The model under review builds one solid part; all positions refer to its coordinate system, in mm. Coordinates: 2 decimals unless noted, no trailing zeros. Order: outer loops, then holes, each group sorted by start corner. A loop starts at its lowest first (then second) coordinate and runs counter-clockwise, first axis right, second up.
```python
from build123d import *

# Parameters (mm, degrees)
SKETCH1_W           = 55.928846154
SKETCH1_H           = 3.175
SKETCH1_W_2         = 3.175
SKETCH1_W_3         = 59.103846154
SKETCH1_H_2         = 26.307142857
SKETCH1_H_3         = 26.307142858
BOSS_EXTRUDE1_DEPTH = 6.35
SKETCH2_W           = 3.175
SKETCH2_H           = 12.7
CUT_EXTRUDE1_DEPTH  = 396.105756412
SKETCH3_W           = 59.103846153
SKETCH3_H           = 3.175
SKETCH3_W_2         = 59.103846154
SKETCH3_W_3         = 3.175
SKETCH3_H_2         = 26.307142857
BOSS_EXTRUDE2_DEPTH = 6.35


with BuildPart() as part:
    # Sketch1 → Boss-Extrude1 (new body)
    with BuildSketch(Plane(origin=(0, 0, 0), x_dir=(1, 0, 0), z_dir=(0, 1, 0))):
        Polygon((0, -88.9), (0, 88.9), (-29.551923077, 88.9), (-88.655769231, 88.9), (-147.759615385, 88.9), (-206.863461538, 88.9), (-265.967307692, 88.9), (-325.071153846, 88.9), (-381, 88.9), (-381, 65.767857143), (-381, 39.460714286), (-381, 13.153571429), (-381, -13.153571429), (-381, -39.460714286), (-381, -65.767857143), (-381, -88.9), (-325.071153846, -88.9), (-265.967307692, -88.9), (-206.863461538, -88.9), (-147.759615385, -88.9), (-88.655769231, -88.9), (-29.551923077, -88.9), align=None)
        Polygon((29.551923077, 88.9), (0, 88.9), (0, -88.9), (29.551923077, -88.9), (88.655769231, -88.9), (147.759615385, -88.9), (206.863461538, -88.9), (265.967307692, -88.9), (325.071153846, -88.9), (381, -88.9), (381, -65.767857143), (381, -39.460714286), (381, -13.153571429), (381, 13.153571429), (381, 39.460714286), (381, 65.767857143), (381, 88.9), (325.071153846, 88.9), (265.967307692, 88.9), (206.863461538, 88.9), (147.759615385, 88.9), (88.655769231, 88.9), align=None)
        with Locations((-353.035576923, -90.4875)):
            Rectangle(SKETCH1_W, SKETCH1_H)
        with Locations((-382.5875, -90.4875)):
            Rectangle(SKETCH1_W_2, SKETCH1_H)
        with Locations((-236.415384615, -90.4875)):
            Rectangle(SKETCH1_W_3, SKETCH1_H)
        with Locations((-382.5875, -52.614285714)):
            Rectangle(SKETCH1_W_2, SKETCH1_H_2)
        with Locations((-118.207692308, -90.4875)):
            Rectangle(SKETCH1_W_3, SKETCH1_H)
        with Locations((-382.5875, 0)):
            Rectangle(SKETCH1_W_2, SKETCH1_H_3)
        with Locations((-382.5875, 52.614285714)):
            Rectangle(SKETCH1_W_2, SKETCH1_H_2)
        with Locations((-382.5875, 90.4875)):
            Rectangle(SKETCH1_W_2, SKETCH1_H)
        with Locations((-353.035576923, 90.4875)):
            Rectangle(SKETCH1_W, SKETCH1_H)
        with Locations((-236.415384615, 90.4875)):
            Rectangle(SKETCH1_W_3, SKETCH1_H)
        with Locations((-118.207692308, 90.4875)):
            Rectangle(SKETCH1_W_3, SKETCH1_H)
        Polygon((-29.551923077, 88.9), (0, 88.9), (29.551923077, 88.9), (29.551923077, 92.075), (-29.551923077, 92.075), align=None)
        with Locations((118.207692308, 90.4875)):
            Rectangle(SKETCH1_W_3, SKETCH1_H)
        Polygon((29.551923077, -88.9), (0, -88.9), (-29.551923077, -88.9), (-29.551923077, -92.075), (29.551923077, -92.075), align=None)
        with Locations((118.207692308, -90.4875)):
            Rectangle(SKETCH1_W_3, SKETCH1_H)
        with Locations((236.415384615, -90.4875)):
            Rectangle(SKETCH1_W_3, SKETCH1_H)
        with Locations((236.415384615, 90.4875)):
            Rectangle(SKETCH1_W_3, SKETCH1_H)
        with Locations((382.5875, 90.4875)):
            Rectangle(SKETCH1_W_2, SKETCH1_H)
        with Locations((382.5875, 52.614285714)):
            Rectangle(SKETCH1_W_2, SKETCH1_H_2)
        with Locations((382.5875, 0)):
            Rectangle(SKETCH1_W_2, SKETCH1_H_3)
        with Locations((382.5875, -52.614285714)):
            Rectangle(SKETCH1_W_2, SKETCH1_H_2)
        with Locations((382.5875, -90.4875)):
            Rectangle(SKETCH1_W_2, SKETCH1_H)
        with Locations((354.623076923, -90.4875)):
            Rectangle(SKETCH1_W_3, SKETCH1_H)
        with Locations((354.623076923, 90.4875)):
            Rectangle(SKETCH1_W_3, SKETCH1_H)
    extrude(amount=BOSS_EXTRUDE1_DEPTH)

    # Sketch2 → Cut-Extrude1 (cut, through all)
    with BuildSketch(Plane(origin=(0, 6.35, 0), x_dir=(1, 0, 0), z_dir=(0, 1, 0))):
        with Locations((-123.03125, 82.55)):
            Rectangle(SKETCH2_W, SKETCH2_H)
        with Locations((-123.03125, -82.55)):
            Rectangle(SKETCH2_W, SKETCH2_H)
        with Locations((130.96875, 82.55)):
            Rectangle(SKETCH2_W, SKETCH2_H)
        with Locations((130.96875, -82.55)):
            Rectangle(SKETCH2_W, SKETCH2_H)
    extrude(amount=-CUT_EXTRUDE1_DEPTH, mode=Mode.SUBTRACT)

    # Sketch3 → Boss-Extrude2 (add)
    with BuildSketch(Plane(origin=(0, 6.35, 0), x_dir=(1, 0, 0), z_dir=(0, 1, 0))):
        with Locations((-177.311538462, -90.4875)):
            Rectangle(SKETCH3_W, SKETCH3_H)
        with Locations((-59.103846154, -90.4875)):
            Rectangle(SKETCH3_W_2, SKETCH3_H)
        with Locations((59.103846154, -90.4875)):
            Rectangle(SKETCH3_W_2, SKETCH3_H)
        with Locations((177.311538462, -90.4875)):
            Rectangle(SKETCH3_W, SKETCH3_H)
        with Locations((382.5875, -26.307142858)):
            Rectangle(SKETCH3_W_3, SKETCH3_H_2)
        with Locations((382.5875, 26.307142858)):
            Rectangle(SKETCH3_W_3, SKETCH3_H_2)
        with Locations((-382.5875, -26.307142858)):
            Rectangle(SKETCH3_W_3, SKETCH3_H_2)
        with Locations((-382.5875, 26.307142858)):
            Rectangle(SKETCH3_W_3, SKETCH3_H_2)
        with Locations((-177.311538462, 90.4875)):
            Rectangle(SKETCH3_W, SKETCH3_H)
        with Locations((-59.103846154, 90.4875)):
            Rectangle(SKETCH3_W_2, SKETCH3_H)
        with Locations((59.103846154, 90.4875)):
            Rectangle(SKETCH3_W_2, SKETCH3_H)
        with Locations((177.311538462, 90.4875)):
            Rectangle(SKETCH3_W, SKETCH3_H)
    extrude(amount=-BOSS_EXTRUDE2_DEPTH)


solid = part.part
```
(1) We need section A-A, the plane x = -293.5. Write out the cut boundary in (y, z).
A:
outline: (0, -88.9) - (6.35, -88.9) - (6.35, 88.9) - (0, 88.9) - close
(2) For pin 1 Ø1.9 at (y, z) = (1.5, -81.5) entering from +X; pin 2 Ø4 at (x, z) = (263, -48) entering from -Y; pin 3 Ø3 at (y, z) = (3, -72.5) entering from -X, all flat-tipped, find the tip position at first contact; note any pin that passes through.
A:
pin 1: stops at x = 381
pin 2: stops at y = 0
pin 3: stops at x = -381
(3) Wall thickness on probe 1 along X at (y, z) = (4.5, 77); probe 2 along X at (y, z) = (5.75, 72.5): over which ranges is each line inside the solid? List them lowest first.
A:
probe 1: x = -381 to -124.62, -121.44 to 129.38, 132.56 to 381
probe 2: x = -381 to 381
